Source: three-view drawing plus pictorial views. Frame: mm from the lowest corner of the part. Round coordinates to 2 decimals unless told otherwise and drop trailing zeros. Order: outer loops, then holes, each group sorted by start corner. A loop starts at its lowest first (then second) coordinate and runs counter-clockwise, first axis right, second up. Notation, with made-up numbers: M 77.5,81.5 L 136.5,81.5 A20 ccw 136.5,102.5 Z; hole C -4,52.25 d11. An arc over 180 degrees is marked long. Return JSON: item names as keys, results as strings. Group by question number.
Q1. Cut plane B-B on y = 22.75. Output: boundary loops of the cut face in (x, z), and give its area (3 significant figures).
Q2. Ray query, probe 1 along Y at (x, z) = (0.7, 5.5). Return the intervals inside material, ascending.
Q3. Cut plane C-C on z = 23. Output: boundary loops of the cut face in (x, y).
Q4. Cut plane A-A on x = 2.25. Output: boundary loops of the cut face in (y, z), and give its area (3 significant figures).
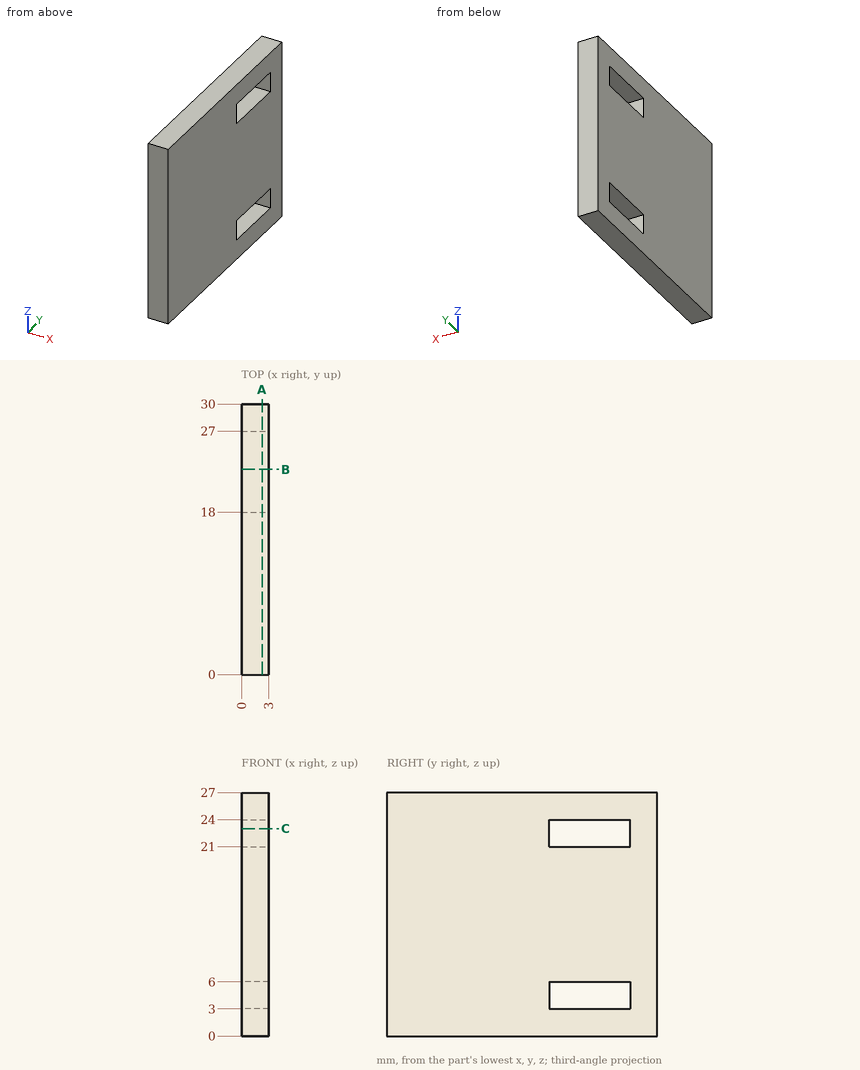
Result sheet:
{
 "1": {"outline": "M 0,0 L 3,0 L 3,3 L 0,3 Z; M 0,6 L 3,6 L 3,21 L 0,21 Z; M 0,24 L 3,24 L 3,27 L 0,27 Z", "area": "63.0 mm²"},
 "2": {"probe 1": "y = 0 to 18, 27 to 30"},
 "3": {"outline": "M 0,0 L 3,0 L 3,18 L 0,18 Z; M 0,27 L 3,27 L 3,30 L 0,30 Z"},
 "4": {"outline": "M 0,0 L 30,0 L 30,27 L 0,27 Z; hole M 18,3 L 27,3 L 27,6 L 18,6 Z; hole M 18,21 L 27,21 L 27,24 L 18,24 Z", "area": "756 mm²"}
}
